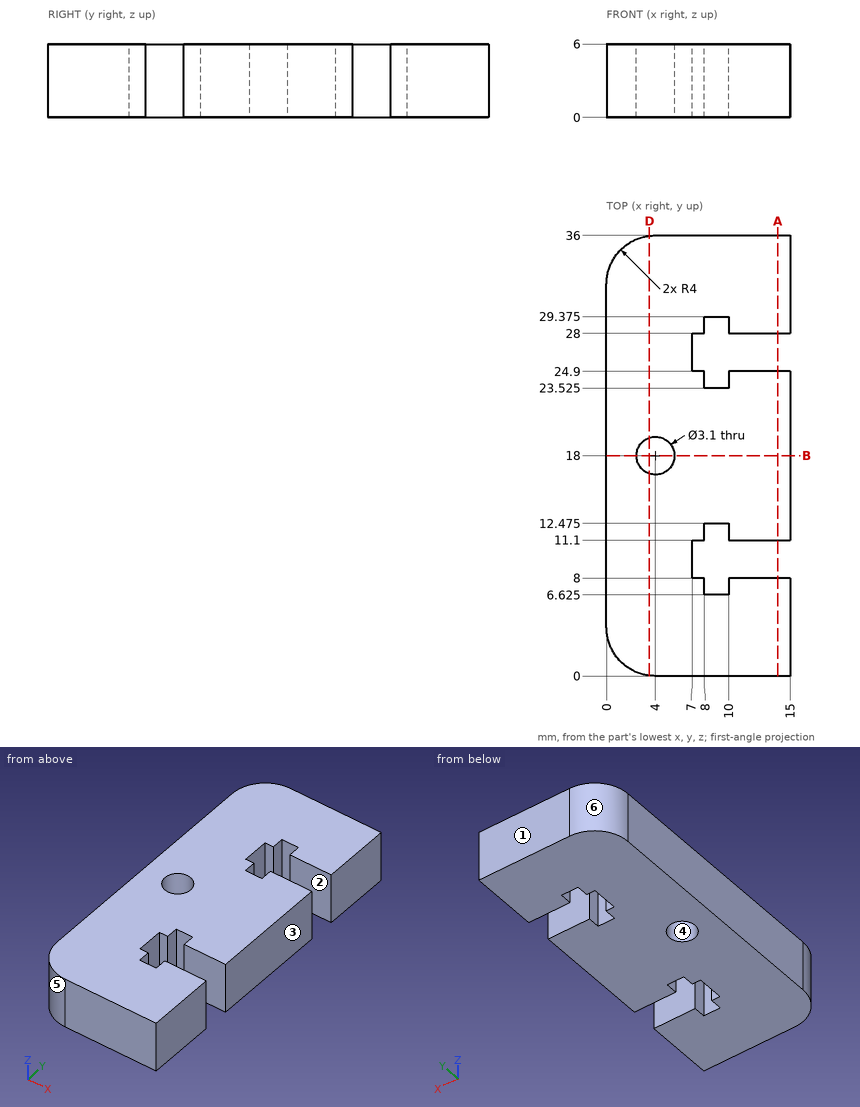
Can you work these out from the drawing? Everything is in mm from the part's minimum corner. A direction names the side the tool comes from. Coordinates: 2 decimals unless noted, no trailing zeros. Loops run counter-clockwise (first coordinate to the right, second up) from the corner with the lowest first, then second, coordinate; pieces in that order, holes last.
1) Imagine slicing it at D-D (x = 3.5). List the corners of the cut face in (y, z) for me.
Reported:
outline: (0.03, 0) - (16.53, 0) - (16.53, 6) - (0.03, 6) - close; (19.47, 0) - (35.97, 0) - (35.97, 6) - (19.47, 6) - close
2) Which directions (+Z, -Z, +X, -X, +Y, -Y) give clear straight access to the entire face, cutting with the end or side of a thin tool? Please do the marked faces 1 and 2.
Reported:
face 1: +Z, -Z, +X, -X, +Y
face 2: +Z, -Z, +X
3) Thinking about a two-plate mould opening in Y: for the marked faces 3, 4, 5 and 6, which applies, released by +Y, released by -Y, zero draft, split by the parting line, or undercut?
Reported:
face 3: zero draft
face 4: undercut
face 5: released by -Y
face 6: released by +Y
4) Please list where these lines run through material, in increasing order: line 1 along Y through (x, z) = (10.5, 5.35); line 2 along Y through (x, z) = (9, 2.15) (3 decimals); line 3 along X through (y, z) = (18, 4.15).
Reported:
line 1: y = 0 to 8, 11.1 to 24.9, 28 to 36
line 2: y = 0 to 6.625, 12.475 to 23.525, 29.375 to 36
line 3: x = 0 to 2.45, 5.55 to 15
5) Imagine slicing it at A-A (x = 14). List the corners of the cut face in (y, z) for me, and give its area (3 significant figures).
Reported:
outline: (0, 0) - (8, 0) - (8, 6) - (0, 6) - close; (11.1, 0) - (24.9, 0) - (24.9, 6) - (11.1, 6) - close; (28, 0) - (36, 0) - (36, 6) - (28, 6) - close
area: 179 mm2
6) Imagine slicing it at B-B (y = 18). List the corners of the cut face in (x, z) for me, and give its area (3 significant figures).
Reported:
outline: (0, 0) - (2.45, 0) - (2.45, 6) - (0, 6) - close; (5.55, 0) - (15, 0) - (15, 6) - (5.55, 6) - close
area: 71.4 mm2
